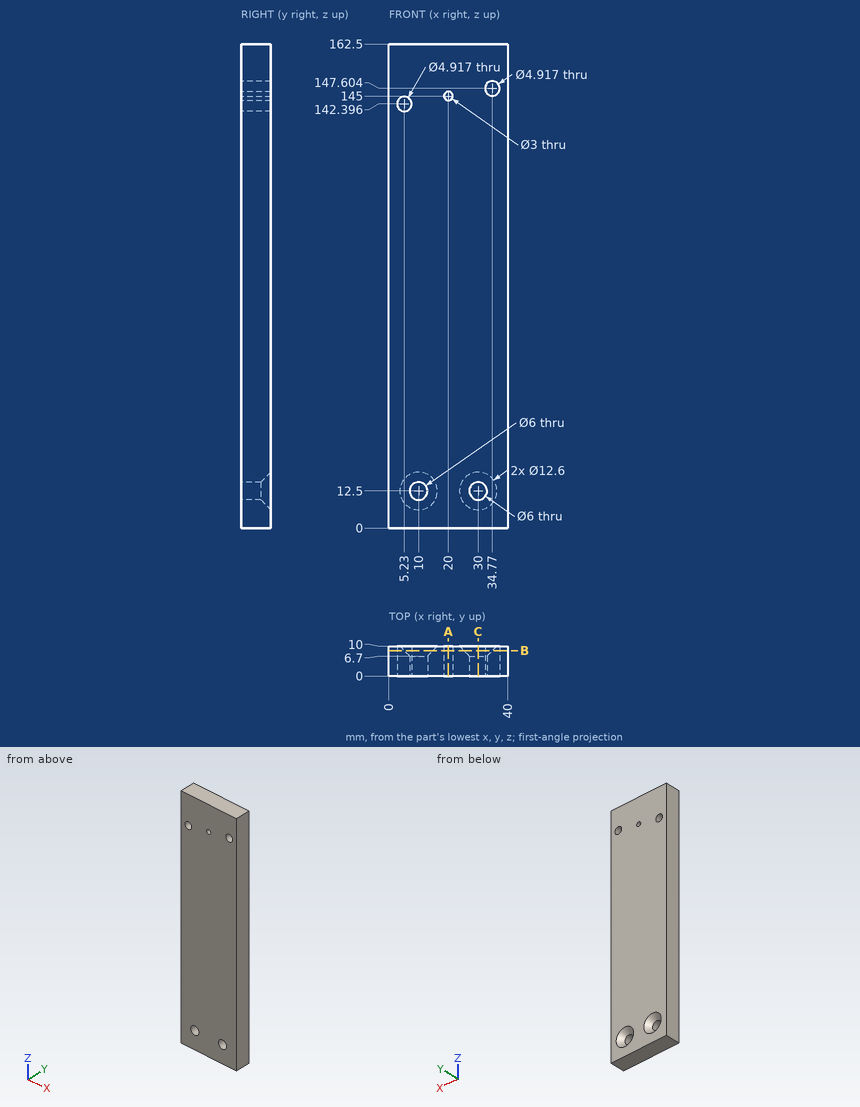
Here's the drawing with two shaded views (mm, measured from the low corner). I have some questions. Coordinates: 2 decimals unless noted, no trailing zeros. Write each loop counter-clockwise with the first axis right and the second up, starting at its lowest first coordinate (ties: lowest second). Pieces come first, ordered by that corner, then holes.
Item 1: Will this pin go through, and if not, where does the flat tip stop? pin 1 (3 mm diameter, centred on x = 5.23, z = 142.4, fed in from -Y).
Item 2: I want a section at B-B on y = 8.5. Write out the boundary of the cut face in (x, z), and give its area (3 significant figures).
Item 3: If I drill on line 1 (Z direction, x = 10, y = 4.5); line 2 (X direction, y = 7.25, z = 145); line 3 (Z direction, x = 5.23, y = 5.5), over which ranges is the centre line in solid material (lowest first)?
Item 4: I want a section at A-A on x = 20. Write out the boundary of the cut face in (y, z), and give its area (4 significant figures).
Item 5: I want a section at C-C on x = 30. Write out the boundary of the cut face in (y, z), and give its area (3 significant figures).
Findings below:
1. pin 1: passes through
2. outline: (0, 0) - (40, 0) - (40, 162.5) - (0, 162.5) - close; hole circle Ø4.92 at (5.23, 142.4); hole circle Ø9.6 at (10, 12.5); hole circle Ø3 at (20, 145); hole circle Ø9.6 at (30, 12.5); hole circle Ø4.92 at (34.77, 147.6)
2. area: 6,310 mm2
3. line 1: z = 0 to 9.5, 15.5 to 162.5
3. line 2: x = 0 to 18.5, 21.5 to 40
3. line 3: z = 0 to 139.94, 144.85 to 162.5
4. outline: (0, 0) - (10, 0) - (10, 143.5) - (0, 143.5) - close; (0, 146.5) - (10, 146.5) - (10, 162.5) - (0, 162.5) - close
4. area: 1,595 mm2
5. outline: (0, 0) - (10, 0) - (10, 6.2) - (6.7, 9.5) - (0, 9.5) - close; (0, 15.5) - (6.7, 15.5) - (10, 18.8) - (10, 162.5) - (0, 162.5) - close
5. area: 1,550 mm2
